Autodesk Inventor part; units mm, degrees
ref_plane "YZ Plane" through (0, 0, 0) normal (1, 0, 0) x (0, 1, 0)
ref_plane "XZ Plane" through (0, 0, 0) normal (0, 1, 0) x (-1, 0, 0)
ref_plane "XY Plane" through (0, 0, 0) normal (0, 0, 1) x (1, 0, 0)
sketch "Sketch1" plane through (0, 0, 0) normal (0, 1, 0) x (-1, 0, 0)
  line L0 (21.35, -20.15) -> (-21.35, -20.15)
  line L1 (-21.35, -20.15) -> (-21.35, 20.15)
  line L2 (-21.35, 20.15) -> (21.35, 20.15)
  line L3 (21.35, 20.15) -> (21.35, -20.15)
  circle A0 centre (-13.3, -15.1) radius 1.65
  circle A1 centre (11.7, -15.1) radius 1.65
  circle A2 centre (-13.3, 15.1) radius 1.65
  circle A3 centre (11.7, 15.1) radius 1.65
  point P0 (0, 0)
  point P1 (0, -20.15)
  point P2 (21.35, 0)
  dimension "d0" = 40.3
  dimension "d1" = 42.7
  dimension "d2" = 6.4
  dimension "d3" = 3.3
  dimension "d4" = 3.4
  dimension "d7" = 25
  dimension "d10" = 30.2
extrude "Extrusion1" add sketch "Sketch1" along normal blind 3.3
sketch "Sketch2" plane through (0, 3.3, 0) normal (0, 1, 0) x (1, 0, 0)
  line L0 (-21.35, 20.15) -> (-21.35, -20.15)
  line L1 (-21.35, -20.15) -> (21.35, -20.15)
  line L2 (-21.35, 20.15) -> (-18.2, 20.15)
  line L3 (-18.2, 20.15) -> (-18.2, -20.15)
  line L4 (-18.2, -20.15) -> (-21.35, -20.15)
  line L5 (-21.35, -20.15) -> (-21.35, 20.15)
  point P0 (0, 0)
  dimension "d15" = 3.15
extrude "Extrusion2" add sketch "Sketch2" along normal blind 42.7
sketch "Sketch3" plane through (-21.35, 0, -20.15) normal (-1, 0, 0) x (0, 0, 1)
  line L0 (40.3, 3.3) -> (40.3, 46)
  line L1 (0, 3.3) -> (0, 46)
  arc A0 (40.3, 25.85) -> (0, 25.85) centre (20.15, 25.85) ccw
  line L2 (0, 46) -> (40.3, 46)
  point P0 (20.15, 0)
  point P1 (20.15, 46)
  point P2 (0, 31.0213)
  point P3 (40.3, 31.0213)
extrude "Extrusion3" cut sketch "Sketch3" against normal through all
sketch "Sketch4" plane through (-21.35, 0, -20.15) normal (-1, 0, 0) x (0, 0, 1)
  arc A0 (26.15, 33.4) -> (14.15, 33.4) centre (20.15, 33.4) ccw
  line L0 (14.15, 33.4) -> (14.15, 18.6)
  line L1 (26.15, 33.4) -> (26.15, 18.6)
  arc A1 (14.15, 18.6) -> (26.15, 18.6) centre (20.15, 18.6) ccw
  arc A2 (40.3, 25.85) -> (0, 25.85) centre (20.15, 25.85) ccw
  point P0 (20.15, 0)
  point P1 (20.15, 46)
  point P2 (20.15, 39.4)
  point P3 (20.15, 46)
  point P4 (20.15, 12.6)
  dimension "d20" = 6.6
  dimension "d21" = 6
  dimension "d22" = 26.8
extrude "Extrusion4" cut sketch "Sketch4" against normal through all
properties part number "Drive Motor Stand"
Read the model definition and answer for the solid it produces. Units are mm, in the model's axes. A direction names the side the tool comes from. Coordinates: 2 decimals unless noted, no trailing zeros. Write each loop counter-clockwise with the first axis right and the second up, starting at its lowest first coordinate (ties: lowest second). Pieces come first, ordered by that corner, then holes. Notation, with made-up numbers: (14, -39.75) - (66, -39.75) arc R33 ccw to (66, -10.75) - close; hole circle Ø5 at (87, -14.75). An arc over 180 degrees is marked (long way). Answer as a JSON object with one key per item and string values. Group by question number.
1. Each of these flat-tipped pins is pushed along its axis until it touches: P1, Ø10, axis at y = 35, z = -16, coming from the +X side; P2, Ø0.9, axis at x = -19.5, y = 29.5, coming from the +Z side; P3, Ø12, axis at x = 5.5, z = -2.5, coming from the +Y side. Where does it stop, or does it pass through?
2. A cutting plane is placed at C-C (y = 32.5). Determine the outline of the cut face in (x, z).
3. A cutting plane is placed at D-D (z = 15.1). Determine the outline of the cut face in (x, y), plus the area to 3 significant figures.
4. The mould has two halves that part along X. Classify faces 1 (the flat face through (-21.35, 12, 0)), 2 (the cylindrical face through (11.776, 1.627, -14.468)), 3 (the flat face through (-6, 3, -20.15)), 4 (the flat face through (-18.2, 15, -5)): +X half, -X half, draft (parallel to the pull), parting line (faces both ways), or undercut.
5. Which of the six approach directions +Z, -Z, +X, -X, +Y, -Y give full straight-line access (tool end or side, diameter ignored) to faces 5 (the flat face through (2, 3.3, 0)), 6 (the flat face through (-20, 26, -6)), 7 (the flat face through (-6, 3, 20.15))?
6. Consider L1, parallel to Z at x = 13.3, y = 1.65; L2, parallel to X at y = 1, z = -15; L3, parallel to Z at x = -11, y = 1. Determine where each line is inside the solid, lowest interval first. Write a range as [from, to].
7. A cutting plane is placed at A-A (x = 13.3). Determine the outline of the cut face in (y, z), plus the area to 3 significant figures.
8. A cutting plane is placed at B-B (z = 0). Determine the outline of the cut face in (x, y), plus the area to 3 significant figures.
Worked out:
{
 "1": {"P1": "stops at x = -18.2", "P2": "stops at z = 19.89", "P3": "stops at y = 3.3"},
 "2": {"outline": "(-21.35, -19.02) - (-18.2, -19.02) - (-18.2, -6) - (-21.35, -6) - close; (-21.35, 6) - (-18.2, 6) - (-18.2, 19.02) - (-21.35, 19.02) - close"},
 "3": {"outline": "(-21.35, 0) - (-13.35, 0) - (-13.35, 3.3) - (-18.2, 3.3) - (-18.2, 39.19) - (-21.35, 39.19) - close; (-10.05, 0) - (11.65, 0) - (11.65, 3.3) - (-10.05, 3.3) - close; (14.95, 0) - (21.35, 0) - (21.35, 3.3) - (14.95, 3.3) - close", "area": "232 mm²"},
 "4": {"face 1": "-X half", "face 2": "undercut", "face 3": "draft", "face 4": "+X half"},
 "5": {"face 5": "+Z, -Z, +X, +Y", "face 6": "+X, -X", "face 7": "+Z, +X, -X, +Y, -Y"},
 "6": {"L1": "z = [-20.15, -16.75], [-13.45, 13.45], [16.75, 20.15]", "L2": "x = [-21.35, -13.35], [-10.05, 11.65], [14.95, 21.35]", "L3": "z = [-20.15, -16.59], [-13.61, 13.61], [16.59, 20.15]"},
 "7": {"outline": "(0, -20.15) - (3.3, -20.15) - (3.3, -16.75) - (0, -16.75) - close; (0, -13.45) - (3.3, -13.45) - (3.3, 13.45) - (0, 13.45) - close; (0, 16.75) - (3.3, 16.75) - (3.3, 20.15) - (0, 20.15) - close", "area": "111 mm²"},
 "8": {"outline": "(-21.35, 0) - (21.35, 0) - (21.35, 3.3) - (-18.2, 3.3) - (-18.2, 12.6) - (-21.35, 12.6) - close; (-21.35, 39.4) - (-18.2, 39.4) - (-18.2, 46) - (-21.35, 46) - close", "area": "191 mm²"}
}
